```python
from build123d import *

# Parameters (mm, degrees)
BOSS_EXTRU_1_DEPTH      = 450
ESQUISSE3_R             = 63.5
ENL_V_MAT_EXTRU_1_DEPTH = 25.4
ESQUISSE4_R             = 25
ENL_V_MAT_EXTRU_2_DEPTH = 20
ESQUISSE2_R             = 50
ENL_V_MAT_EXTRU_3_DEPTH = 97
COQUE1_T                = -30


with BuildPart() as part:
    # Esquisse1 → Boss.-Extru.1 (new body)
    with BuildSketch(Plane.XY):
        Polygon((75, 129.903810568), (375, 129.903810568), (450, 0), (0, 0), align=None)
    extrude(amount=BOSS_EXTRU_1_DEPTH)

    # Esquisse3 → Enlèv. mat.-Extru.1 (cut)
    with BuildSketch(Plane(origin=(0, 129.903810568, 0), x_dir=(1, 0, 0), z_dir=(0, 1, 0))):
        with Locations(Location((225, -225, 0), (0, 0, 270))):
            Circle(ESQUISSE3_R)
    extrude(amount=-ENL_V_MAT_EXTRU_1_DEPTH, mode=Mode.SUBTRACT)

    # Esquisse4 → Enlèv. mat.-Extru.2 (cut)
    with BuildSketch(Plane(origin=(0, 104.503810568, 0), x_dir=(1, 0, 0), z_dir=(0, 1, 0))):
        with Locations(Location((225, -225, 0), (0, 0, 270))):
            Circle(ESQUISSE4_R)
    extrude(amount=-ENL_V_MAT_EXTRU_2_DEPTH, mode=Mode.SUBTRACT)

    # Esquisse2 → Enlèv. mat.-Extru.3 (cut)
    with BuildSketch(Plane.XZ):
        with Locations(Location((225, 225, 0), (0, 0, 270))):
            Circle(ESQUISSE2_R)
    extrude(amount=-ENL_V_MAT_EXTRU_3_DEPTH, mode=Mode.SUBTRACT)

    # Coque1
    coque1_openings = [part.faces().sort_by_distance(p)[0] for p in [
        (443.636038969, 0, 225),
    ]]
    offset(amount=COQUE1_T, openings=coque1_openings, kind=Kind.INTERSECTION)


solid = part.part
```
Design review of the part built by this model. Coordinates are the model's own, in mm. A direction names the side the tool comes from. Round coordinates to 2 decimals unless told otherwise and drop trailing zeros. Write each loop counter-clockwise with the first axis right and the second up, starting at its lowest first coordinate (ties: lowest second). Pieces come first, ordered by that corner, then holes.
Item 1: We need section D-D on y = 85. Write out the cut boundary in (x, z).
Item 2: We need section B-B on y = 47. Write out the cut boundary in (x, z).
Item 3: For probe 1 along Z at (x, y) = (167, 43.5); probe 2 along Z at (x, y) = (259, 41); probe 3 along X at (y, z) = (28.5, 163.5), list the stretches that pass through material, from the lowest coordinate up.
Item 4: We need section A-A on x = 225. Write out the cut boundary in (y, z).
Item 5: Clearance check with flat-ended pins moving along their axes: pin 1 Ø3 at (y, z) = (58.5, 125.5) entering from +X; pin 2 Ø1.5 at (x, z) = (52.5, 301.5) entering from +Y; pin 3 Ø5 at (y, z) = (27.5, 337) entering from +X. State where each tip first meets the part, or that it passes through.
Item 6: The part is to be moulded in two halves that separate along Z. For faces 1 (the flat face through (228, 66, 450)), 2 (the flat face through (189.6, 129.904, 171.9)), 3 (the cylindrical face through (154.03, 36.73, 188.08)), say which applies: +Z half, -Z half, draft (parallel to the pull), parting line (faces both ways), or undercut.
Item 7: We need section C-C on z = 225. Write out the cut boundary in (x, y), and give its area (3 significant figures).
Item 8: For faces 4 (the flat face through (228, 66, 0)), 5 (the flat face through (267, 74.504, 294)), 6 (the flat face through (198, 104.504, 224)), list the 3-axis set-ups (+Z, -Z, +X, -X, +Y, -Y) from which the entire face can be reached by the end or side of a thin tool; tool diameter is ignored.
Returned:
1. outline: (49.07, 0) - (400.93, 0) - (400.93, 450) - (49.07, 450) - close; circle Ø187 at (225, 225); hole (83.72, 30) - (366.28, 30) - (366.28, 420) - (83.72, 420) - close; hole circle Ø100 at (225, 225)
2. outline: (27.14, 0) - (422.86, 0) - (422.86, 450) - (27.14, 450) - close; circle Ø160 at (225, 225); hole (61.78, 30) - (388.22, 30) - (388.22, 420) - (61.78, 420) - close; hole circle Ø100 at (225, 225)
3. probe 1: z = 0 to 30, 169.9 to 280.1, 420 to 450
3. probe 2: z = 0 to 30, 152.58 to 188.34, 261.66 to 297.42, 420 to 450
3. probe 3: x = 16.45 to 51.1, 173.84 to 276.16, 398.9 to 433.55
4. outline: (0, 0) - (129.9, 0) - (129.9, 161.5) - (104.5, 161.5) - (104.5, 200) - (97, 200) - (97, 175) - (0, 175) - (0, 145) - (74.5, 145) - (74.5, 131.5) - (99.9, 131.5) - (99.9, 30) - (0, 30) - close; (0, 275) - (97, 275) - (97, 250) - (104.5, 250) - (104.5, 288.5) - (129.9, 288.5) - (129.9, 450) - (0, 450) - (0, 420) - (99.9, 420) - (99.9, 318.5) - (74.5, 318.5) - (74.5, 305) - (0, 305) - close
5. pin 1: stops at x = 417.09
5. pin 2: stops at y = 92.23
5. pin 3: stops at x = 435.57
6. face 1: +Z half
6. face 2: draft
6. face 3: undercut
7. outline: (0, 0) - (34.64, 0) - (92.32, 99.9) - (131.5, 99.9) - (131.5, 74.5) - (145, 74.5) - (145, 0) - (175, 0) - (175, 97) - (200, 97) - (200, 104.5) - (161.5, 104.5) - (161.5, 129.9) - (75, 129.9) - close; (250, 97) - (275, 97) - (275, 0) - (305, 0) - (305, 74.5) - (318.5, 74.5) - (318.5, 99.9) - (357.68, 99.9) - (415.36, 0) - (450, 0) - (375, 129.9) - (288.5, 129.9) - (288.5, 104.5) - (250, 104.5) - close
7. area: 19,800 mm2
8. face 4: -Z, +X, -X, +Y, -Y
8. face 5: -Y
8. face 6: +Y
